```python
from build123d import *

# Parameters (mm, degrees)
SKETCH1_W           = 4
SKETCH1_H           = 40
BOSS_EXTRUDE1_DEPTH = 39
SKETCH2_W           = 4
SKETCH2_H           = 12
CUT_EXTRUDE1_DEPTH  = 39
SKETCH5_R           = 3.567899071
CUT_EXTRUDE3_DEPTH  = 12
FILLET6_R           = 2
FILLET7_R           = 2


with BuildPart() as part:
    # Sketch1 → Boss-Extrude1 (new body)
    with BuildSketch(Plane.XY):
        with Locations((-2, 5.490763705)):
            Rectangle(SKETCH1_W, SKETCH1_H)
    extrude(amount=BOSS_EXTRUDE1_DEPTH)

    # Sketch2 → Cut-Extrude1 (cut)
    with BuildSketch(Plane(origin=(0, 0, 0), x_dir=(0, 0, -1), z_dir=(1, 0, 0))):
        with Locations((-2, 19.490763705)):
            Rectangle(SKETCH2_W, SKETCH2_H)
    extrude(amount=-CUT_EXTRUDE1_DEPTH, mode=Mode.SUBTRACT)

    # Sketch5 → Cut-Extrude3 (cut)
    with BuildSketch(Plane(origin=(0, 25.490763705, 0), x_dir=(1, 0, 0), z_dir=(0, 1, 0))):
        with Locations((-2, -1.249948334)):
            Circle(SKETCH5_R)
    extrude(amount=-CUT_EXTRUDE3_DEPTH, mode=Mode.SUBTRACT)

    # Fillet6
    fillet6_edges = [part.edges().sort_by_distance(p)[0] for p in [
        (-2, 25.490763705, 39),
    ]]
    fillet(fillet6_edges, radius=FILLET6_R)

    # Fillet7
    fillet7_edges = [part.edges().sort_by_distance(p)[0] for p in [
        (-2, -14.509236295, 0),
        (-2, -14.509236295, 39),
    ]]
    fillet(fillet7_edges, radius=FILLET7_R)


solid = part.part
```
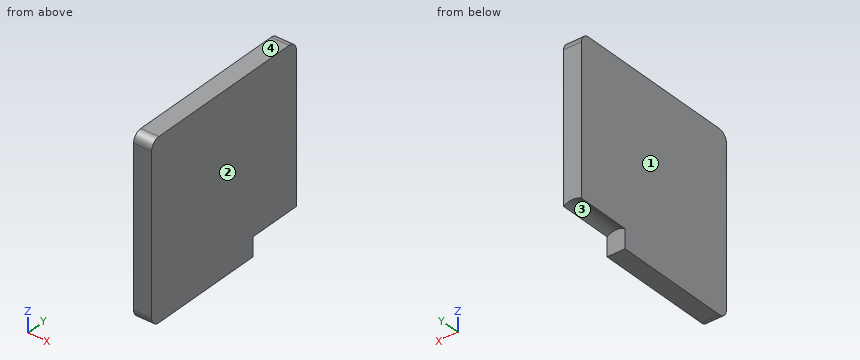
Check sheet for the modelled part. Datum: model origin and axes. Units: mm. Face numbers are marked on the shaded views. Round coordinates to 2 decimals unless told otherwise and drop trailing zeros. Order: outer loops, then holes, each group sorted by start corner. A loop starts at its lowest first (then second) coordinate and runs counter-clockwise, first axis right, second up. Notation, with made-up numbers: (74.5, 82) -> (79.5, 82) arc R32 ccw to (79.5, 110) -> close; hole circle Ø9 at (-9, 68.5). An arc over 180 degrees is marked (long way). Use CSV: the item, a comma, the result in double quotes.
(1) Depth check by flat-ended pin: pin 1 (8 mm diameter, centred on y = 11, z = 31.5, fed in from +X). Enter the tip coordinate at first touch or a pass-through.
Worked out:
pin 1,"x = 0"
(2) Cross-section at C-C (x = -0.55). Record the boundary of the cut face in (y, z).
Worked out:
outline,"(-14.51, 2) arc R2 ccw to (-12.51, 0) -> (13.49, 0) -> (13.49, 4.51) -> (25.49, 4.51) -> (25.49, 37) arc R2 ccw to (23.49, 39) -> (-12.51, 39) arc R2 ccw to (-14.51, 37) -> close"
(3) Cross-section at A-A (x = -2.9). Record the boundary of the cut face in (y, z), and give its area (3 significant figures).
Worked out:
outline,"(-14.51, 2) arc R2 ccw to (-12.51, 0) -> (13.49, 0) -> (13.49, 4.7) -> (25.49, 4.7) -> (25.49, 37) arc R2 ccw to (23.49, 39) -> (-12.51, 39) arc R2 ccw to (-14.51, 37) -> close"
area,"1,500 mm²"
(4) Cross-section at B-B (y = 21). Record the boundary of the cut face in (x, z).
Worked out:
outline,"(-4, 4.2) arc R3.57 cw to (0, 4.2) -> (0, 39) -> (-4, 39) -> close"
(5) Material ranges on line 1 along Z through (x, y) = (-3.6, 19.5); line 2 along Z through (x, y) = (-2.05, 14), recorded low to high. Write a range as from..to.
Worked out:
line 1,"4.44..39"
line 2,"4.82..39"
(6) Draft check along X on the marked faces 1, 2, 3 and 4. Enter one of: pulls with the +X half, pulls with the -X half, needs draft (parallel to the pull), parting line crosses it, or undercut.
Worked out:
face 1,"pulls with the -X half"
face 2,"pulls with the +X half"
face 3,"undercut"
face 4,"needs draft"
